Autodesk Inventor part; units mm, degrees
ref_plane "YZ Plane" through (0, 0, 0) normal (1, 0, 0) x (0, 1, 0)
ref_plane "XZ Plane" through (0, 0, 0) normal (0, 1, 0) x (-1, 0, 0)
ref_plane "XY Plane" through (0, 0, 0) normal (0, 0, 1) x (1, 0, 0)
sketch "Эскиз1" plane through (0, 0, 0) normal (0, 1, 0) x (-1, 0, 0)
  line L0 (0, 0) -> (-5, 0)
  line L1 (-5, 0) -> (-5, -20)
  line L2 (-5, -20) -> (0, -20)
  line L3 (0, -20) -> (0, 0)
  dimension "d0" = 5
  dimension "d1" = 20
extrude "Выдавливание1" add sketch "Эскиз1" along normal blind 7
sketch "Эскиз2" plane through (0, 7, 0) normal (0, 1, 0) x (1, 0, 0)
  line L0 (0, 0) -> (5, 0)
  line L1 (5, 0) -> (5, 20)
  line L2 (5, 20) -> (0, 20)
  line L3 (0, 20) -> (0, 0)
  line L4 (0, 0) -> (5, 0)
  line L5 (5, 0) -> (15, 0)
  line L6 (15, 0) -> (15, 20)
  line L7 (15, 20) -> (5, 20)
  line L8 (5, 20) -> (5, 0)
  dimension "d4" = 10
  dimension "d5" = 20
extrude "Выдавливание2" add sketch "Эскиз2" along normal blind 3
chamfer "Фаска1" distance 2 angle 45 1 edges at (5, 7, -10)
sketch "Эскиз3" plane through (0, 0, 0) normal (0, 0, 1) x (1, 0, 0)
  line L0 (0, 0) -> (25, 0)
  line L1 (25, 0) -> (25, 3)
  line L2 (25, 3) -> (0, 3)
  line L3 (0, 3) -> (0, 0)
  line L4 (0, 0) -> (5, 0) construction
  line L5 (5, 0) -> (5, 5) construction
  line L6 (7, 7) -> (5, 5) construction
  line L7 (7, 7) -> (15, 7) construction
  line L8 (15, 7) -> (15, 10) construction
  line L9 (0, 10) -> (15, 10) construction
  line L10 (0, 0) -> (0, 10) construction
  line L11 (0, 3) -> (5, 3)
  line L12 (5, 3) -> (5, 13)
  line L13 (5, 13) -> (0, 13)
  line L14 (0, 13) -> (0, 3)
  line L15 (5, 13) -> (15, 13)
  line L16 (15, 13) -> (15, 10)
  line L17 (15, 10) -> (5, 10)
  line L18 (5, 10) -> (5, 13)
  line L19 (0, 0) -> (5, 0)
  line L20 (0, 0) -> (-10, 0)
  line L21 (-10, 0) -> (-10, 3)
  line L22 (-10, 3) -> (0, 3)
  line L23 (0, 3) -> (0, 0)
  line L24 (0, 13) -> (-10, 13)
  line L25 (-10, 13) -> (-10, 10)
  line L26 (-10, 10) -> (0, 10)
  line L27 (0, 10) -> (0, 13)
  line L28 (0, 13) -> (3, 10)
  line L29 (0, 10) -> (15, 10)
  line L30 (-1.6585, 10) -> (0, 8.3415)
  line L31 (0, 0) -> (0, 10)
  point P0 (0, 8.3415)
  dimension "d11" = 3
  dimension "d12" = 25
  dimension "d13" = 5
  dimension "d14" = 10
  dimension "d15" = 10
  dimension "d16" = 3
  dimension "d17" = 10
  dimension "d18" = 3
extrude "Выдавливание3" add sketch "Эскиз3" against normal blind 20 contours L20 L21 L22 L3 | L30 L26 L14 | L26 L25 L24 L14 | L14 L28 L29
properties part number "test_support2"
Geometry: final body of the model. Coordinates: model frame, mm. A direction names the side the tool comes from. Coordinates: 2 decimals unless noted, no trailing zeros. Order: outer loops, then holes, each group sorted by start corner. A loop starts at its lowest first (then second) coordinate and runs counter-clockwise, first axis right, second up. Notation, with made-up numbers: (22.5, 18) - (48.5, 18) arc R20 ccw to (48.5, 36) - close; hole circle Ø2 at (-35, 6). An arc over 180 degrees is marked (long way). Return JSON: item names as keys, results as strings. Group by question number.
1. Cut plane C-C (x = 7.5). Output: boundary loops of the cut face in (y, z).
2. Material intervals for line 1 along Y through (x, z) = (-6.75, -11); line 2 along X through (y, z) = (4.75, -9.5); line 3 along X through (y, z) = (8.25, -3.25), sorted ascending. Write a range as [from, to].
3. Set-up query: faces 4 (the face through (-0.84, 9.18, -9.86)), 5 (the face through (-10, 12, -10)), 6 (the face through (9, 10, -10)), 7 (the face through (5, 2, -10)). Return all of +Z, -Z, +X, -X, +Y, -Y with unobstructed straight access to the full face (end or side cutting, diameter ignored); none if empty.
4. Pin query (flat end, axial travel): pin 1 (2 mm diameter, centred on x = 8.5, z = -8, fed in from +Y); pin 2 (4 mm diameter, centred on x = 10.5, z = -6.5, fed in from -Y); pin 3 (1.5 mm diameter, centred on y = 7.5, z = -11.5, fed in from -X). Return the tip coordinate at first contact, or that it passes through.
5. Cut plane B-B (z = -6.25). Output: boundary loops of the cut face in (x, y), plus the area to 3 significant figures.
6. Cut plane D-D (y = 2). Output: boundary loops of the cut face in (x, z).
7. Cut plane A-A (x = -5.5). Output: boundary loops of the cut face in (y, z), plus the area to 3 significant figures.
8. Pull-direction query (Y, two-part tool) for faces 1 (the face through (-5, 3, -10)), 2 (the face through (11, 7, -10)), 3 (the face through (3, 6, -20)); classes: pulls with the +Y half, pulls with the -Y half, needs draft (parallel to the pull), parting line crosses it, or undercut.
Resolved:
{
 "1": {"outline": "(7, -20) - (10, -20) - (10, 0) - (7, 0) - close"},
 "2": {"line 1": "y = [0, 3], [10, 13]", "line 2": "x = [0, 5]", "line 3": "x = [0, 15]"},
 "3": {"face 4": "+Z, -Z, -X", "face 5": "+Z, -Z, -X, +Y, -Y", "face 6": "+Z, -Z, +X, +Y", "face 7": "+Z, -Z, +X, -Y"},
 "4": {"pin 1": "stops at y = 10", "pin 2": "stops at y = 7", "pin 3": "stops at x = 0"},
 "5": {"outline": "(-10, 0) - (5, 0) - (5, 5) - (7, 7) - (15, 7) - (15, 10) - (3, 10) - (0, 13) - (-10, 13) - (-10, 10) - (-1.66, 10) - (0, 8.34) - (0, 3) - (-10, 3) - close", "area": "148 mm²"},
 "6": {"outline": "(-10, -20) - (5, -20) - (5, 0) - (-10, 0) - close"},
 "7": {"outline": "(0, -20) - (3, -20) - (3, 0) - (0, 0) - close; (10, -20) - (13, -20) - (13, 0) - (10, 0) - close", "area": "120 mm²"},
 "8": {"face 1": "undercut", "face 2": "pulls with the -Y half", "face 3": "needs draft"}
}
